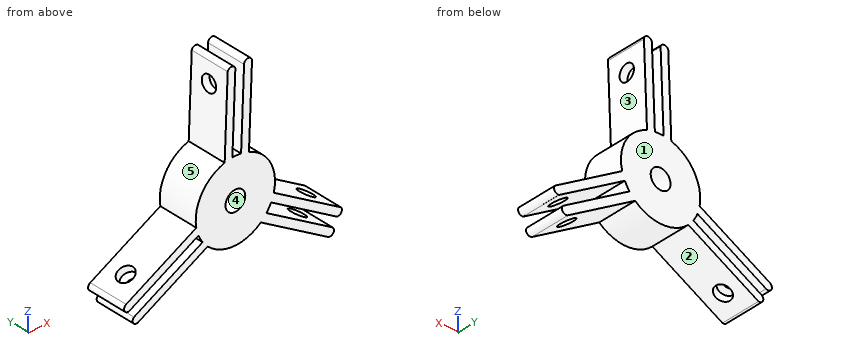
from build123d import *

# Parameters (mm, degrees)
SKETCH1_R           = 2.5
BOSS_EXTRUDE1_DEPTH = 10
SKETCH2_R           = 2
CUT_EXTRUDE1_DEPTH  = 10
CIRPATTERN1_COUNT   = 3


with BuildPart() as part:
    # Sketch1 → Boss-Extrude1 (new body)
    with BuildSketch(Plane(origin=(0, 0, 0), x_dir=(1, 0, 0), z_dir=(0, 1, 0))):
        with BuildLine():
            Line((3.42943918, -9.393558799), (4.197898245, -29.378790113))
            ThreePointArc((4.197898245, -29.378790113), (3.237059632, -30.416474632), (2.199375114, -29.455636019))
            Line((2.199375114, -29.455636019), (1.447231615, -9.894721858))
            ThreePointArc((1.447231615, -9.894721858), (0.350023332, -9.993872306), (-0.751433173, -9.971727442))
            Line((-0.751433173, -9.971727442), (0.000999669, -29.540166516))
            ThreePointArc((0.000999669, -29.540166516), (-0.935779597, -30.318112399), (-1.929530696, -29.614398009))
            Line((-1.929530696, -29.614398009), (-2.697989761, -9.629166695))
            ThreePointArc((-2.697989761, -9.629166695), (-8.461744243, -5.329060364), (-9.849780142, 1.726797949))
            Line((-9.849780142, 1.726797949), (-27.541727692, 11.053908534))
            ThreePointArc((-27.541727692, 11.053908534), (-27.959969541, 12.404861441), (-26.609016634, 12.823103289))
            Line((-26.609016634, 12.823103289), (-9.2926963, 3.694021585))
            ThreePointArc((-9.2926963, 3.694021585), (-8.829958965, 4.693807055), (-8.260052699, 5.636623938))
            Line((-8.260052699, 5.636623938), (-25.58303447, 14.769217519))
            ThreePointArc((-25.58303447, 14.769217519), (-25.788365734, 15.969465103), (-24.682055646, 16.478221605))
            Line((-24.682055646, 16.478221605), (-6.990108095, 7.15111102))
            ThreePointArc((-6.990108095, 7.15111102), (-0.384229532, 9.992615657), (6.420340962, 7.66676085))
            Line((6.420340962, 7.66676085), (23.343829448, 18.324881579))
            ThreePointArc((23.343829448, 18.324881579), (24.722909908, 18.011613191), (24.40964152, 16.63253273))
            Line((24.40964152, 16.63253273), (7.845464685, 6.200700273))
            ThreePointArc((7.845464685, 6.200700273), (8.479935633, 5.300065251), (9.011485871, 4.335103505))
            Line((9.011485871, 4.335103505), (25.582034801, 14.770948997))
            ThreePointArc((25.582034801, 14.770948997), (26.724145331, 14.348647296), (26.611586342, 13.136176404))
            Line((26.611586342, 13.136176404), (9.688097856, 2.478055676))
            ThreePointArc((9.688097856, 2.478055676), (8.845973775, -4.663555293), (3.42943918, -9.393558799))
        make_face()
        Circle(SKETCH1_R, mode=Mode.SUBTRACT)
    extrude(amount=BOSS_EXTRUDE1_DEPTH)

    # Sketch2 → Cut-Extrude1 (cut)
    with BuildSketch(Plane(origin=(3.063714471, 0, -0.117803948), x_dir=(-0.038422953, 0, -0.999261566), z_dir=(0.999261566, 0, -0.038422953))):
        with Locations((-24.518391454, 5)):
            Circle(SKETCH2_R)
    cut_extrude1 = extrude(amount=-CUT_EXTRUDE1_DEPTH, mode=Mode.SUBTRACT)

    # CirPattern1: Cut-Extrude1 ×3 about axis
    cirpattern1_axis = Axis((0, 10, 0), (0, -1, 0))
    for i in range(1, CIRPATTERN1_COUNT):
        add(cut_extrude1.rotate(cirpattern1_axis, i * 360 / CIRPATTERN1_COUNT), mode=Mode.SUBTRACT)


solid = part.part
Build history of the part. All positions in model axes, mm. Face numbers are marked on the shaded views. A direction names the side the tool comes from. Round coordinates to 2 decimals unless told otherwise and drop trailing zeros. Write each loop counter-clockwise with the first axis right and the second up, starting at its lowest first coordinate (ties: lowest second). Pieces come first, ordered by that corner, then holes. Notation, with made-up numbers: (73, 71) -> (103, 71) arc R34 ccw to (103, 103) -> close; hole circle Ø3 at (49.25, 67). An arc over 180 degrees is marked (long way). Write item = value, one per line.
(1) Tool access for the marked faces 1 and 2: list every direction of +Z, -Z, +X, -X, +Y, -Y with a clear straight run to the whole face (end or side of a thin tool).
Answer:
face_1 = +Z, -Z, +X, -X, +Y
face_2 = -Z, +Y, -Y
(2) Band-saw the part on B-B (x = 11). Give the cut face in (y, z).
Answer:
outline = (0, -10.55) -> (10, -10.55) -> (10, -8.19) -> (0, -8.19) -> close; (0, -5.59) -> (10, -5.59) -> (10, -3.3) -> (0, -3.3) -> close
(3) Probe L1, parallel to X at y = 7, z = 0; L2, parallel to Z at x = 11, y = 3; L3, parallel to X at y = 8.5, z = -7. List the from-to ranges inside material, lowest first.
Answer:
L1 = -10 to -2.5, 2.5 to 10
L2 = -10.55 to -8.19, -5.59 to -3.3
L3 = -19.85 to -15.56, -10.85 to 9.11, 13.24 to 16.87
(4) Band-saw the part on D-D (y = 6.25). State how many separate pieces and enclosed holes the cut face has, then the cut area to 3 significant figures.
Answer:
separate_pieces = 7
enclosed_holes = 1
area = 499 mm2
(5) Band-saw the part on A-A (z = 0). Give the cut face in (x, y).
Answer:
outline = (-10, 0) -> (-2.5, 0) -> (-2.5, 10) -> (-10, 10) -> close; (2.5, 0) -> (10, 0) -> (10, 10) -> (2.5, 10) -> close
(6) Two-plate mould, pull along X, no slides. Class the marked faces 3, 4 and 5: pulls with the +X half, pulls with the -X half, needs draft (parallel to the pull), parting line crosses it, or undercut.
Answer:
face_3 = pulls with the +X half
face_4 = undercut
face_5 = pulls with the -X half
(7) Flat gauge pins, fed straight in: pin 1 (4 mm diameter, centred on y = 1.5, z = 13.5, fed in from -X); pin 2 (2 mm diameter, centred on x = -3.5, y = 5.5, fed in from -Z); pin 3 (3 mm diameter, centred on y = 4, z = 11, fed in from +X). Where does each tip first touch, or does it go through?
Answer:
pin_1 = -2.63
pin_2 = -9.68
pin_3 = 3.55
(8) Band-saw the part on C-C (y = 2). Give the cut face in (x, z).
Answer:
outline = (-27.54, -11.05) arc R1 ccw to (-26.61, -12.82) -> (-9.29, -3.69) arc R10 ccw to (-8.26, -5.64) -> (-25.58, -14.77) arc R1 ccw to (-24.68, -16.48) -> (-6.99, -7.15) arc R10 ccw to (6.42, -7.67) -> (23.34, -18.32) arc R1 ccw to (24.41, -16.63) -> (7.85, -6.2) arc R10 ccw to (9.01, -4.34) -> (25.58, -14.77) arc R1 ccw to (26.61, -13.14) -> (9.69, -2.48) arc R10 ccw to (3.43, 9.39) -> (4.2, 29.38) arc R1 ccw to (2.2, 29.46) -> (1.45, 9.89) arc R10 ccw to (-0.75, 9.97) -> (0, 29.54) arc R1 ccw to (-1.93, 29.61) -> (-2.7, 9.63) arc R10 ccw to (-9.85, -1.73) -> close; hole circle Ø5 at (0, 0)
